CAD build for the part. Positions are in the model's coordinates, mm. A direction names the side the tool comes from. Give positions to 0.01 mm unless a question says otherwise; leave off trailing zeros. Write each loop counter-clockwise with the first axis right and the second up, starting at its lowest first coordinate (ties: lowest second). Pieces come first, ordered by that corner, then holes. Notation, with made-up numbers: (37.5, -23.5) -> (62.5, -23.5) arc R25 ccw to (62.5, 15.5) -> close; hole circle Ø2 at (47.25, 0). An arc over 180 degrees is marked (long way). Answer as a JSON object with one key per item and string values.
```python
from build123d import *

# Parameters (mm, degrees)
BOSS_EXTRUDE1_DEPTH = 1.5
SKETCH2_R           = 4
SKETCH2_R_2         = 1.6
CUT_EXTRUDE1_DEPTH  = 2.5
SKETCH3_W           = 26
SKETCH3_H           = 1.5
BOSS_EXTRUDE4_DEPTH = 31.5
SKETCH4_R           = 5
SKETCH4_R_2         = 2
CUT_EXTRUDE2_DEPTH  = 34
FILLET1_R           = 1.5


with BuildPart() as part:
    # Sketch1 → Boss-Extrude1 (new body)
    with BuildSketch(Plane.XY):
        with BuildLine():
            Line((0, 0), (26, 0))
            Line((26, 0), (26, 20))
            ThreePointArc((26, 20), (13, 33), (0, 20))
            Line((0, 20), (0, 0))
        make_face()
    extrude(amount=BOSS_EXTRUDE1_DEPTH)

    # Sketch2 → Cut-Extrude1 (cut, through all)
    with BuildSketch(Plane(origin=(0, 0, 0), x_dir=(-1, 0, 0), z_dir=(0, 0, -1))):
        with Locations((-13, 20)):
            Circle(SKETCH2_R)
        with Locations((-21.5, 20)):
            Circle(SKETCH2_R_2)
        with Locations((-4.5, 20)):
            Circle(SKETCH2_R_2)
    extrude(amount=-CUT_EXTRUDE1_DEPTH, mode=Mode.SUBTRACT)

    # Sketch3 → Boss-Extrude4 (add)
    with BuildSketch(Plane(origin=(0, 0, 0), x_dir=(-1, 0, 0), z_dir=(0, 0, -1))):
        with Locations((-13, 0.75)):
            Rectangle(SKETCH3_W, SKETCH3_H)
    extrude(amount=BOSS_EXTRUDE4_DEPTH)

    # Sketch4 → Cut-Extrude2 (cut, through all)
    with BuildSketch(Plane.XZ):
        with Locations((13, -15.75)):
            Circle(SKETCH4_R)
        with Locations((5, -8.75)):
            Circle(SKETCH4_R_2)
        with Locations((21, -8.75)):
            Circle(SKETCH4_R_2)
        with Locations((21, -22.75)):
            Circle(SKETCH4_R_2)
        with Locations((5, -22.75)):
            Circle(SKETCH4_R_2)
    extrude(amount=-CUT_EXTRUDE2_DEPTH, mode=Mode.SUBTRACT)

    # Fillet1
    fillet1_edges = [part.edges().sort_by_distance(p)[0] for p in [
        (26, 0.75, -31.5),
        (0, 0.75, -31.5),
    ]]
    fillet(fillet1_edges, radius=FILLET1_R)


solid = part.part
```
1) Slice it at B-B (z = -8.75). List the corners of the cut face in (x, y).
Model answer:
{"outline": "(0, 0) -> (3, 0) -> (3, 1.5) -> (0, 1.5) -> close; (7, 0) -> (19, 0) -> (19, 1.5) -> (7, 1.5) -> close; (23, 0) -> (26, 0) -> (26, 1.5) -> (23, 1.5) -> close"}
2) Wall check: probe 1 along Z at (x, y) = (21, 0.9); probe 2 along Y at (x, z) = (13, 0.7); probe 3 along Z at (x, y) = (15, 27). Give the ranges that are in metal, low to high.
Model answer:
{"probe 1": "z = -31.5 to -24.75, -20.75 to -10.75, -6.75 to 1.5", "probe 2": "y = 0 to 16, 24 to 33", "probe 3": "z = 0 to 1.5"}
3) Slice it at C-C (y = 21). List the corners of the cut face in (x, z).
Model answer:
{"outline": "(0.04, 0) -> (3.25, 0) -> (3.25, 1.5) -> (0.04, 1.5) -> close; (5.75, 0) -> (9.13, 0) -> (9.13, 1.5) -> (5.75, 1.5) -> close; (16.87, 0) -> (20.25, 0) -> (20.25, 1.5) -> (16.87, 1.5) -> close; (22.75, 0) -> (25.96, 0) -> (25.96, 1.5) -> (22.75, 1.5) -> close"}
4) Mould opens along Z. For faces 1 (the flat face through (26, 1, -10)), 2 (the flat face through (13, 14, 0)), 3 (the cylindrical face through (15.307, 0.74, -20.186)), 4 (the cylindrical face through (3.526, 0.74, -7.398)) say: released by +Z, released by -Z, zero draft, split by the parting line, or undercut.
Model answer:
{"face 1": "zero draft", "face 2": "released by -Z", "face 3": "undercut", "face 4": "undercut"}
5) Slice it at A-A (x = 13). List the corners of the cut face in (y, z), then the cut area to 4 significant figures.
Model answer:
{"outline": "(0, -31.5) -> (1.5, -31.5) -> (1.5, -20.75) -> (0, -20.75) -> close; (0, -10.75) -> (1.5, -10.75) -> (1.5, 0) -> (16, 0) -> (16, 1.5) -> (0, 1.5) -> close; (24, 0) -> (33, 0) -> (33, 1.5) -> (24, 1.5) -> close", "area": "69.75 mm2"}
6) 3-axis set-ups, long thin cutter, end or side, ignore diameter. For faces 5 (the flat face through (7, 1.5, -16)), 6 (the cylindrical face through (19.526, 0.74, -21.398)): which of +Z, -Z, +X, -X, +Y, -Y reach the whole face in a straight line?
Model answer:
{"face 5": "-Z, +X, -X, +Y", "face 6": "+Y, -Y"}
7) Slice it at D-D (x = 4). List the corners of the cut face in (y, z), then the cut area to 3 significant figures.
Model answer:
{"outline": "(0, -31.5) -> (1.5, -31.5) -> (1.5, -24.48) -> (0, -24.48) -> close; (0, -21.02) -> (1.5, -21.02) -> (1.5, -10.48) -> (0, -10.48) -> close; (0, -7.02) -> (1.5, -7.02) -> (1.5, 0) -> (18.48, 0) -> (18.48, 1.5) -> (0, 1.5) -> close; (21.52, 0) -> (29.38, 0) -> (29.38, 1.5) -> (21.52, 1.5) -> close", "area": "76.4 mm2"}
8) Pin check, flat tips, straight feed: pin 1 (9 mm diameter, centred on x = 13, y = 20, fed in from -Z); pin 2 (9 mm diameter, centred on x = 13, z = -15.75, fed in from +Y); pin 3 (8 mm diameter, centred on x = 14.5, z = -18, fed in from +Y); pin 4 (6.5 mm diameter, centred on x = 5, z = -8.75, fed in from -Y). Stop position of each tip, or through.
Model answer:
{"pin 1": "stops at z = 0", "pin 2": "passes through", "pin 3": "stops at y = 1.5", "pin 4": "stops at y = 0"}
